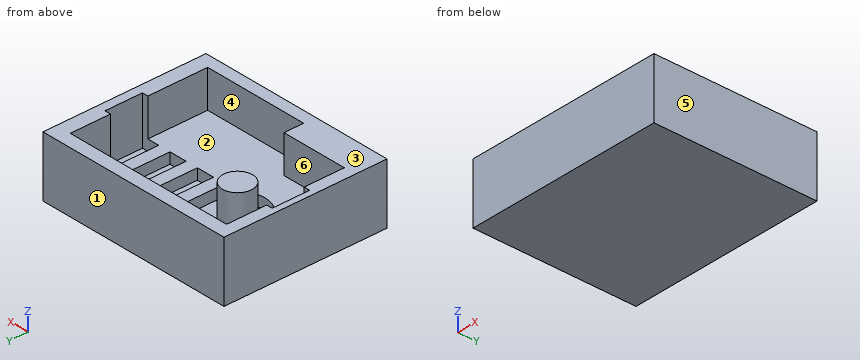
from build123d import *

# Parameters (mm, degrees)
PAD004_DEPTH             = 8.2
SKETCH014_W              = 28.5
SKETCH014_H              = 6.2
PAD005_DEPTH             = 1.8
SKETCH015_R              = 2.9
POCKET004_DEPTH          = 0.6
SKETCH016_W              = 2.05
SKETCH016_H              = 6.2
POCKET005_DEPTH          = 1.8
CLONE012_PLACEMENT_ANGLE = 180
BOX_W                    = 33
BOX_H                    = 27
BOX_DEPTH                = 10
SKETCH_W                 = 3
SKETCH_H                 = 3.25
POCKET009_DEPTH          = 6.2
SKETCH021_W              = 1
SKETCH021_H              = 6.2
POCKET010_DEPTH          = 8
SKETCH022_R              = 4.55
POCKET011_DEPTH          = 1.8
SKETCH023_R              = 2.5
PAD_DEPTH                = 6


with BuildPart() as body011:
    # Sketch013 → Pad004 (new body)
    with BuildSketch(Plane.XY):
        with BuildLine():
            Line((0, 0), (28.5, 0))
            Line((28.5, 0), (28.5, 22.75))
            Line((28.5, 22.75), (14, 22.75))
            Line((14, 22.75), (14, 22.5))
            ThreePointArc((11, 19.5), (13.12132, 20.37868), (14, 22.5))
            Line((11, 19.5), (0, 19.5))
            Line((0, 19.5), (0, 0))
        make_face()
    extrude(amount=PAD004_DEPTH)

    # Sketch014 (on Face9 of Pad004) → Pad005 (join)
    with BuildSketch(Plane.XY.offset(8.2)):
        with Locations((14.25, 9.75)):
            Rectangle(SKETCH014_W, SKETCH014_H)
    extrude(amount=PAD005_DEPTH)

    # Sketch015 (on Face11 of Pad005) → Pocket004 (cut)
    with BuildSketch(Plane.XY.offset(10)):
        with Locations((8.735056, 9.75)):
            Circle(SKETCH015_R)
    extrude(amount=-POCKET004_DEPTH, mode=Mode.SUBTRACT)

    # Sketch016 (on Face10 of Pocket004) → Pocket005 (cut)
    with BuildSketch(Plane.XY.offset(10)):
        with Locations((15.5, 9.75)):
            Rectangle(SKETCH016_W, SKETCH016_H)
        Polygon((21.525, 12.85), (21.525, 6.65), (19.475, 6.65), (19.475, 12.85), (20.5, 12.85), align=None)
        with Locations((25.5, 9.75)):
            Rectangle(SKETCH016_W, SKETCH016_H)
    extrude(amount=-POCKET005_DEPTH, mode=Mode.SUBTRACT)


with BuildPart() as body011_1:
    # Clone012 placement: moved
    add(body011.part.moved(Location((0, 22.75, 12))).rotate(Axis((0, 22.75, 12), (1, 0, 0)), CLONE012_PLACEMENT_ANGLE))


with BuildPart() as model_body012:
    # Box → Box (new body)
    with BuildSketch(Plane(origin=(-2, -2, 0), x_dir=(1, 0, 0), z_dir=(0, 0, 1))):
        with Locations((16.5, 13.5)):
            Rectangle(BOX_W, BOX_H)
    extrude(amount=BOX_DEPTH)

    # Cut: cut Body011
    add(body011_1.part, mode=Mode.SUBTRACT)

    # Sketch (on Face3 of BaseFeature001) → Pocket009 (cut)
    with BuildSketch(Plane.XY.offset(10)):
        with Locations((12.5, 1.625)):
            Rectangle(SKETCH_W, SKETCH_H)
    extrude(amount=-POCKET009_DEPTH, mode=Mode.SUBTRACT)

    # Sketch021 (on Face3 of Pocket009) → Pocket010 (cut)
    with BuildSketch(Plane.XY.offset(10)):
        with Locations((-0.5, 13)):
            Rectangle(SKETCH021_W, SKETCH021_H)
        with Locations((29, 13)):
            Rectangle(SKETCH021_W, SKETCH021_H)
    extrude(amount=-POCKET010_DEPTH, mode=Mode.SUBTRACT)

    # Sketch022 (on Face17 of Pocket010) → Pocket011 (cut)
    with BuildSketch(Plane.XY.offset(3.8)):
        with Locations((8.735056, 13)):
            Circle(SKETCH022_R)
    extrude(amount=-POCKET011_DEPTH, mode=Mode.SUBTRACT)

    # Sketch023 (on Face39 of Pocket011) → Pad (join)
    with BuildSketch(Plane.XY.offset(2)):
        with Locations((8.735056, 13)):
            Circle(SKETCH023_R)
    extrude(amount=PAD_DEPTH)


solid = model_body012.part
Build history of the part. All positions in model axes, mm. Face numbers are marked on the shaded views. A direction names the side the tool comes from. Give positions to 0.01 mm unless a question says otherwise; leave off trailing zeros. Order: outer loops, then holes, each group sorted by start corner. A loop starts at its lowest first (then second) coordinate and runs counter-clockwise, first axis right, second up. Notation, with made-up numbers: M -5,-29.75 L 32,-29.75 A31 ccw 32,-3.75 Z; hole C 58,-0.5 d11. An arc over 180 degrees is marked long. Use one line per item in the form item = value.
1) Saw through at C-C (y = 13). Give the cut face in (x, z) (3 decimals).
Calculated:
outline = M -2,0 L 31,0 L 31,10 L 29.5,10 L 29.5,2 L 26.525,2 L 26.525,3.8 L 24.475,3.8 L 24.475,2 L 21.525,2 L 21.525,3.8 L 19.475,3.8 L 19.475,2 L 16.525,2 L 16.525,3.8 L 14.475,3.8 L 14.475,2 L 11.235,2 L 11.235,8 L 6.235,8 L 6.235,2 L -1,2 L -1,10 L -2,10 Z
2) Saw through at D-D (x = 19). Give the cut face in (y, z).
Calculated:
outline = M -2,0 L 25,0 L 25,10 L 22.75,10 L 22.75,3.8 L 16.1,3.8 L 16.1,2 L 9.9,2 L 9.9,3.8 L 0,3.8 L 0,10 L -2,10 Z
3) Drop flat-ended pins along their axis: pin 1 (1.5 mm diameter, centred on x = 23.5, y = 11.5, fed in from +Z); pin 2 (11.5 mm diameter, centred on x = 12.5, y = 9.5, fed in from +Z). Give the stop position or say it passes through.
Calculated:
pin_1 = 2
pin_2 = 8
4) Probe probe 1 along Y at (x, z) = (20, 9); probe 2 along X at (y, z) = (1.75, 5.25); probe 3 along X at (y, z) = (10.75, 5.5). List the from-to ranges inside material, lowest first.
Calculated:
probe_1 = -2 to 0, 22.75 to 25
probe_2 = -2 to 11, 28.5 to 31
probe_3 = -2 to -1, 7.65 to 9.82, 29.5 to 31
5) Two-plate mould, pull along Y, no slides. Class the marked faces 1, 2, 3 and 4: released by +Y, released by -Y, zero draft, split by the parting line, or undercut.
Calculated:
face_1 = released by +Y
face_2 = undercut
face_3 = zero draft
face_4 = undercut
6) Saw through at A-A (z = 7.25). Give the cut face in (x, y), plus the area to 3 significant figures.
Calculated:
outline = M -2,-2 L 31,-2 L 31,25 L -2,25 Z; C 8.74,13 d5; hole M -1,9.9 L 0,9.9 L 0,3.25 L 11,3.25 L 11,0 L 28.5,0 L 28.5,9.9 L 29.5,9.9 L 29.5,16.1 L 28.5,16.1 L 28.5,22.75 L 0,22.75 L 0,16.1 L -1,16.1 Z
area = 286 mm2
7) Tool access for the marked faces 5 and 6: list every direction of +Z, -Z, +X, -X, +Y, -Y with a clear straight run to the whole face (end or side of a thin tool).
Calculated:
face_5 = +Z, -Z, +X, +Y, -Y
face_6 = +Z
8) Saw through at B-B (x = 3.5). Give the cut face in (y, z), plus the area to 3 significant figures.
Calculated:
outline = M -2,0 L 25,0 L 25,10 L 22.75,10 L 22.75,3.8 L 16.1,3.8 L 16.1,2 L 9.9,2 L 9.9,3.8 L 3.25,3.8 L 3.25,10 L -2,10 Z
area = 138 mm2
